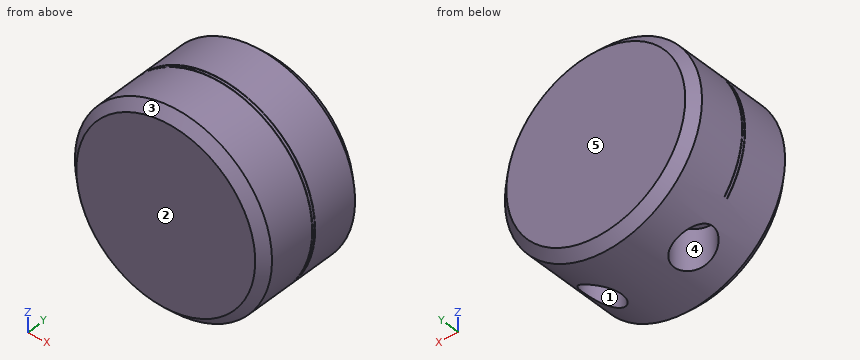
Autodesk Inventor part; units mm, degrees
ref_plane "Work Plane1" through (0, 0, -32.5) normal (0, 0, -1) x (-1, 0, 0)
ref_plane "YZ Plane" through (0, 0, 0) normal (1, 0, 0) x (0, 1, 0)
ref_plane "XZ Plane" through (0, 0, 0) normal (0, 1, 0) x (-1, 0, 0)
sketch "Sketch1" plane through (0, 0, 0) normal (0, 1, 0) x (-1, 0, 0)
  circle A0 centre (0, 0) radius 32.5
  dimension "d0" = 65
extrude "Extrusion1" add sketch "Sketch1" along normal blind 38.5
sketch "Sketch2" plane through (0, 0, 0) normal (0, -1, 0) x (1, 0, 0)
  circle A0 centre (0, 0) radius 25.5
  dimension "d3" = 51
extrude "Extrusion2" add sketch "Sketch2" along normal blind 23.4
chamfer "Chamfer1" distance 3 angle 45 2 edges at (32.5, 38.5, 0) (32.5, 0, 0)
sketch "Sketch3" plane through (0, -23.4, 0) normal (0, -1, 0) x (1, 0, 0)
  line L0 (0, 0) -> (0, -10.5) construction
  circle A0 centre (0, 0) radius 25.5
  line L1 (0, -10.5) -> (5.75, -10.5)
  line L2 (5.75, -10.5) -> (5.75, -24.8433)
  line L3 (0, -10.5) -> (-5.75, -10.5)
  line L4 (-5.75, -10.5) -> (-5.75, -24.8433)
  line L5 (5.75, -24.8433) -> (-5.75, -24.8433)
  line L6 (-15, 15) -> (15, 15) construction
  line L7 (15, 15) -> (15, -15) construction
  line L8 (15, -15) -> (-15, -15) construction
  line L9 (-15, -15) -> (-15, 15) construction
  line L10 (-15, 15) -> (15, -15) construction
  line L11 (15, 15) -> (-15, -15) construction
  line L12 (5.65, 5.65) -> (-5.65, 5.65) construction
  line L13 (-5.65, 5.65) -> (-5.65, -5.65) construction
  line L14 (-5.65, -5.65) -> (5.65, -5.65) construction
  line L15 (5.65, -5.65) -> (5.65, 5.65) construction
  line L16 (5.65, 5.65) -> (-5.65, -5.65) construction
  line L17 (-5.65, 5.65) -> (5.65, -5.65) construction
  dimension "d10" = 10.5
  dimension "d14" = 5.75
  dimension "d15" = 5.75
  dimension "d16" = 30
  dimension "d17" = 30
  dimension "d35" = 11.3
  dimension "d36" = 11.3
hole "Hole1" at (15, -23.4, -15) at (-15, -23.4, -15) at (15, -23.4, 15) at (-15, -23.4, 15) direction (0, 1, 0) diameter 2.5 depth 4 tip angle 118
thread "Thread1"
thread "Thread2"
thread "Thread3"
thread "Thread4"
extrude "Extrusion3" cut sketch "Sketch3" against normal blind 12 contours L5 A0 | L4 L3 L1 L2 L5
hole "Hole2" at (5.65, -23.4, 5.65) at (5.65, -23.4, -5.65) at (-5.65, -23.4, 5.65) at (-5.65, -23.4, -5.65) direction (0, 1, 0) diameter 2.1 depth 3 tip angle 118
thread "Thread5"
thread "Thread6"
thread "Thread7"
thread "Thread8"
ref_plane "Work Plane1" through (0, 0, -32.5) normal (0, 0, -1) x (-1, 0, 0)
sketch "Sketch4" plane through (0, 0, -32.5) normal (0, 0, -1) x (-1, 0, 0)
  line L0 (-25.5, -23.4) -> (25.5, -23.4)
  line L1 (-32.5, 3) -> (32.5, 3)
  line L2 (32.5, 35.5) -> (-32.5, 35.5)
  line L3 (0, -23.4) -> (0, 18.1) construction
  line L4 (32.5, 3) -> (32.5, 35.5)
  line L5 (-32.5, 3) -> (-32.5, 35.5)
  line L6 (32.5, 17.6) -> (32.5, 18.6)
  line L7 (-20, 18.1) -> (20, 18.1) construction
  line L8 (0, 18.1) -> (-15, 18.1)
  line L9 (0, 18.1) -> (15, 18.1)
  circle A0 centre (-15, 18.1) radius 6.35
  circle A1 centre (15, 18.1) radius 6.35
  point P0 (0, 0)
  point P1 (-5.75, -23.4)
  point P2 (5.75, -23.4)
  dimension "d52" = 41.5
  dimension "d53" = 1
  dimension "d54" = 20
  dimension "d56" = 15
  dimension "d57" = 15
  dimension "d58" = 12.7
  dimension "d59" = 12.7
extrude "Extrusion5" cut sketch "Sketch4" against normal blind 15 contours A0 | A1
sketch "Sketch6" plane through (0, 0, 0) normal (1, 0, 0) x (0, 1, 0)
  line L0 (3, 32.5) -> (35.5, 32.5)
  line L1 (35.5, 32.5) -> (19.25, 32.5)
  line L2 (19.25, 32.5) -> (19.75, 32.5)
  line L3 (19.25, 32.5) -> (18.75, 32.5)
  line L4 (18.875, 32.625) -> (18.625, 32.625)
  line L5 (18.625, 32.625) -> (18.625, 32.375)
  line L6 (18.625, 32.375) -> (18.875, 32.375)
  line L7 (18.875, 32.375) -> (18.875, 32.625)
  line L8 (18.875, 32.625) -> (18.625, 32.375) construction
  line L9 (18.625, 32.625) -> (18.875, 32.375) construction
  line L10 (19.875, 32.625) -> (19.625, 32.625)
  line L11 (19.625, 32.625) -> (19.625, 32.375)
  line L12 (19.625, 32.375) -> (19.875, 32.375)
  line L13 (19.875, 32.375) -> (19.875, 32.625)
  line L14 (19.875, 32.625) -> (19.625, 32.375) construction
  line L15 (19.625, 32.625) -> (19.875, 32.375) construction
  line L16 (-35.78, 0) -> (50.88, 0)
  point P0 (0, 0)
  dimension "d83" = 16.25
  dimension "d84" = 0.5
  dimension "d85" = 0.5
  dimension "d86" = 0.25
  dimension "d87" = 0.25
  dimension "d88" = 0.25
  dimension "d89" = 0.25
revolve "Revolution4" cut sketch "Sketch6" angle 250 mid plane about axis through (0, -10, 0) along (0, 1, 0)
ref_plane "Work Plane2" through (0, 0, 0) normal (0, -1, 0) x (1, 0, 0)
split body "Split1" result two bodies by plane through (0, 0, 0) normal (0, -1, 0) first body at (-14.161, -15.6, -20.6026)
split "Split2" plane through (0, 0, 0) removes the side toward (0, -1, 0)
properties part number "SweepV0.991_HEAD_Rev.1" material "LCP Plastic"
Here's how the part is built. I have some questions about the finished solid (model axes, mm). Face numbers are marked on the shaded views. A direction names the side the tool comes from. Round coordinates to 2 decimals unless told otherwise and drop trailing zeros. Order: outer loops, then holes, each group sorted by start corner. A loop starts at its lowest first (then second) coordinate and runs counter-clockwise, first axis right, second up. Notation, with made-up numbers: M -27.75,73.25 L -19.75,73.25 A23 cw -19.75,104.25 Z; hole C 40,-10 d4. An arc over 180 degrees is marked long. Answer as CSV lines item,"result".
Item 1: Which directions (+Z, -Z, +X, -X, +Y, -Y) give clear straight access to the entire face, cutting with the end or side of a thin tool? Please do the marked faces 4 and 5.
From the geometry:
face 4,"-Z"
face 5,"+Z, -Z, +X, -X, +Y"
Item 2: For pin 1 (10 mm diameter, centred on x = 11, z = 3.5, fed in from -Y); pin 2 (10 mm diameter, centred on y = 29.5, z = -14.5, fed in from +X); pin 3 (4 mm diameter, centred on x = -13.5, y = 16, fed in from -Z); pin 4 (6 mm diameter, centred on x = 10, y = 12, fed in from +Z), each with a flat end and sliding along its axis, tell me the tip position at first contact or that it passes through.
From the geometry:
pin 1,"y = 0"
pin 2,"x = 31.08"
pin 3,"z = -17.5"
pin 4,"z = 31.74"
Item 3: We'd pull the mould along X, two halves only. Please class the marked faces 1, 2 and 3: +X half, -X half, draft (parallel to the pull), parting line (faces both ways), or undercut.
From the geometry:
face 1,"undercut"
face 2,"draft"
face 3,"parting line"
Item 4: Imagine slicing it at A-A on y = 34. List the corners of the cut face in (x, z) for me.
From the geometry:
outline,"C 0,0 d65"
Item 5: Please list where these lines run through material, in increasing order: L1, parallel to Y at x = 15, z = -25; L2, parallel to X at y = 18.5, z = -20; L3, parallel to Z at x = 1, y = 9. Write a range as [from, to].
From the geometry:
L1,"[0, 11.75], [24.45, 38.5]"
L2,"[-25.62, -21.34], [-8.66, 8.66], [21.34, 25.62]"
L3,"[-32.48, 32.48]"
